Job drawing, mm, ordinate dimensions from the low corner. One solid piece. A direction names the side the tool comes from. Give positions to 0.01 mm unless a question says otherwise; leave off trailing zeros. Order: outer loops, then holes, each group sorted by start corner. A loop starts at its lowest first (then second) coordinate and runs counter-clockwise, first axis right, second up.
1. Drop flat-ended pins along their axis: pin 1 Ø3 at (y, z) = (5.5, 23) entering from -X; pin 2 Ø8 at (y, z) = (9.5, 15) entering from +X; pin 3 Ø8 at (x, z) = (10.5, 16) entering from -Y. Give the stop position or say it passes through.
2. Probe line 1 (Z direction, x = 12.25, y = 10.25); line 2 (Y direction, x = 7, z = 12.5); line 3 (X direction, y = 9.75, z = 16.5). List the from-to ranges inside material, lowest first.
3. Slice it at D-D on y = 1.5. List the corners of the cut face in (x, z).
4. Slice it at A-A on y = 7. List the corners of the cut face in (x, z), and give its area (3 significant figures).
5. Which spindle directions (+Z, -Z, +X, -X, +Y, -Y) get a long thin tool onto all of the face, cutting with end or side? Do the marked faces 1 and 2. Say none if no direction does.
6. Slice it at C-C on z = 29.5. List the corners of the cut face in (x, y), and give its area (3 significant figures).
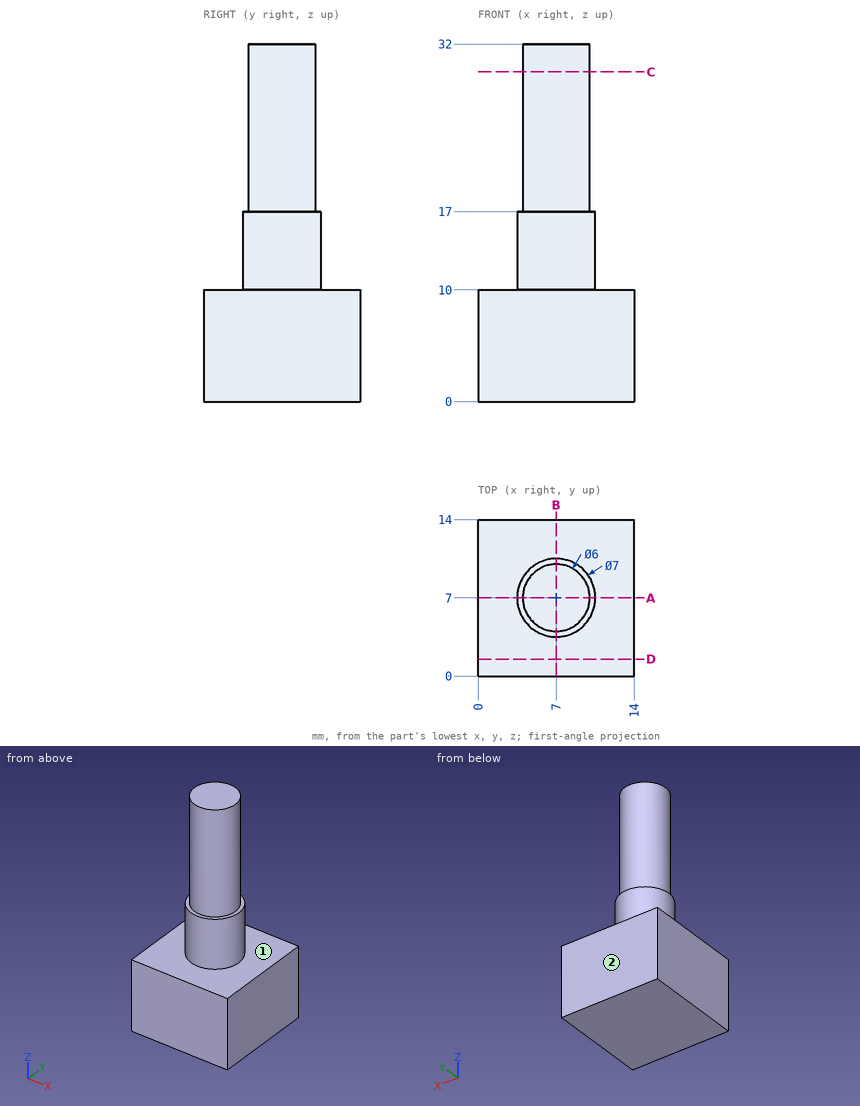
Data:
1. pin 1: stops at x = 4
1. pin 2: stops at x = 10.5
1. pin 3: stops at y = 3.5
2. line 1: z = 0 to 10
2. line 2: y = 3.5 to 10.5
2. line 3: x = 4.83 to 9.17
3. outline: (0, 0) - (14, 0) - (14, 10) - (0, 10) - close
4. outline: (0, 0) - (14, 0) - (14, 10) - (10.5, 10) - (10.5, 17) - (10, 17) - (10, 32) - (4, 32) - (4, 17) - (3.5, 17) - (3.5, 10) - (0, 10) - close
4. area: 279 mm2
5. face 1: +Z
5. face 2: +Z, -Z, +X, -X, +Y
6. outline: circle Ø6 at (7, 7)
6. area: 28.3 mm2
